Source: CAD feature listing. Evaluate the final solid. Frame: model axes, mm. A direction names the side the tool comes from. Round coordinates to 2 decimals unless told otherwise and drop trailing zeros. Order: outer loops, then holes, each group sorted by start corner. A loop starts at its lowest first (then second) coordinate and runs counter-clockwise, first axis right, second up. Notation, with made-up numbers: (-34.5, 9) - (2.5, 9) arc R18 ccw to (2.5, 43) - close; hole circle Ø9 at (-13.5, -24). An arc over 180 degrees is marked (long way). Put each result on its own line as item: value. Start each with the question number.
1) Access query for faces 5 (the face through (-3, 1, 8.6)), 6 (the face through (6, 0, 4)). Directions: +Z, -Z, +X, -X, +Y, -Y. A direction counts if a zero-diameter tool reaches every point of the face in a straight line with its end or side. Return the directions, or none.
2) Section A-A on y = 0. Output: boundary loops of the cut face in (x, z), then the cut area to 3 significant figures.
3) Contact query for flat-ended pins moving along their axis: P1, Ø6, axis at x = -0.5, y = -3.5, coming from the +Z side; P2, Ø3, axis at y = 3.5, z = 16, coming from the +X side. Output: stop coordinate, or through.
4) Line query: probe 1 along Z at (x, y) = (-0.75, -3.5); probe 2 along Y at (x, z) = (0, 16); probe 3 along X at (y, z) = (-2.5, 23.25). Output: solid intervals per line, ascending. Write a range as [from, to].
5) Mould query, pull axis Y, two halves, no side actions, for faces 1 (the face through (0, -6, 4)), 2 (the face through (-3, 0, 17)), 3 (the face through (0, 0, 0)), 4 (the face through (0, 6, 4)). Classes: +Y half, -Y half, draft (parallel to the pull), parting line (faces both ways), or undercut.
6) Section D-D on y = -4.5. Output: boundary loops of the cut face in (x, z).
7) Section C-C on z = 21.5. Output: boundary loops of the cut face in (x, y), then the cut area to 3 significant figures.
```python
from build123d import *

# Parameters (mm, degrees)
BOX012_W          = 12
BOX012_H          = 12
BOX012_DEPTH      = 8.6
CYLINDER003_R     = 3
CYLINDER003_DEPTH = 25


with BuildPart() as part:
    # Box012 → Box012 (join)
    with BuildSketch(Plane(origin=(-6, -6, 0), x_dir=(1, 0, 0), z_dir=(0, 0, 1))):
        with Locations((6, 6)):
            Rectangle(BOX012_W, BOX012_H)
    extrude(amount=BOX012_DEPTH)

    # Cylinder003 → Cylinder003 (join)
    with BuildSketch(Plane.XY):
        Circle(CYLINDER003_R)
    extrude(amount=CYLINDER003_DEPTH)


solid = part.part
```
Answer sheet:
1. face 5: +Z
1. face 6: +Z, -Z, +X, +Y, -Y
2. outline: (-6, 0) - (6, 0) - (6, 8.6) - (3, 8.6) - (3, 25) - (-3, 25) - (-3, 8.6) - (-6, 8.6) - close
2. area: 202 mm^2
3. P1: z = 25
3. P2: x = 2.24
4. probe 1: [0, 8.6]
4. probe 2: [-3, 3]
4. probe 3: [-1.66, 1.66]
5. face 1: -Y half
5. face 2: parting line
5. face 3: draft
5. face 4: +Y half
6. outline: (-6, 0) - (6, 0) - (6, 8.6) - (-6, 8.6) - close
7. outline: circle Ø6 at (0, 0)
7. area: 28.3 mm^2
